Input: part model. Units: mm. Frame: model coordinates. Give positions to 0.01 mm unless a question says otherwise; leave off trailing zeros. Order: outer loops, then holes, each group sorted by start corner. A loop starts at its lowest first (then second) coordinate and runs counter-clockwise, first axis right, second up. Notation, with made-up numbers: (-28, 1.25) - (-16, 1.25) arc R19 cw to (-16, 15.25) - close; hole circle Ø8 at (80.5, 10.25). An arc over 180 degrees is marked (long way). Use a Markdown table: item, result.
Autodesk Inventor part; units mm, degrees
ref_plane "YZ Plane" through (0, 0, 0) normal (1, 0, 0) x (0, 1, 0)
ref_plane "XZ Plane" through (0, 0, 0) normal (0, 1, 0) x (-1, 0, 0)
ref_plane "XY Plane" through (0, 0, 0) normal (0, 0, 1) x (1, 0, 0)
sketch "Sketch2" plane through (0, 0, 0) normal (0, 0, 1) x (1, 0, 0)
  line L0 (0, 0) -> (-9.9, 0)
  line L1 (-4.95, 0) -> (-4.95, 2.5)
  line L2 (-4.95, 0) -> (-2.45, 0) construction
  circle A0 centre (-4.95, 5) radius 2.5
  line L3 (-4.95, 7.5) -> (32.05, 7.5) construction
  line L4 (0, 44.5) -> (0, 0)
  line L5 (0, 0) -> (-9.9, 0)
  line L6 (-9.9, 0) -> (-9.9, 44.5)
  line L7 (0, 45.5) -> (0, 0)
  line L8 (0, 0) -> (-9.9, 0)
  line L9 (-9.9, 0) -> (-9.9, 45.5)
  line L10 (-4.95, 7.5) -> (66.05, 7.5) construction
  line L11 (0, 0) -> (-9.9, 0)
  line L12 (-9.9, 0) -> (-9.9, 81)
  line L13 (-9.9, 81) -> (0, 81)
  line L14 (0, 81) -> (0, 0)
  dimension "d35" = 5
  dimension "d33" = 2.5
  dimension "d34" = 90
  dimension "d46" = 9.9
  dimension "d47" = 81
extrude "Extrusion6" add sketch "Sketch2" along normal blind 5
properties part number "Elbow_Cube_Holder_TestFit_V2"
1. Material intervals for line 1 along Y through (x, z) = (-4.95, 2.65); line 2 along X through (y, z) = (5, 1.35); line 3 along Y through (x, z) = (-7, 1.9), sorted ascending.
Response:
| item | result |
|---|---|
| line 1 | y = 0 to 2.5, 7.5 to 81 |
| line 2 | x = -9.9 to -7.45, -2.45 to 0 |
| line 3 | y = 0 to 3.57, 6.43 to 81 |
2. Section query A-A (x = -4.95). Return loops of the section in (y, z).
Response:
| item | result |
|---|---|
| outline | (0, 0) - (2.5, 0) - (2.5, 5) - (0, 5) - close; (7.5, 0) - (81, 0) - (81, 5) - (7.5, 5) - close |
3. Section query B-B (y = 6.5). Return loops of the section in (x, z), then the cut area to 3 significant figures.
Response:
| item | result |
|---|---|
| outline | (-9.9, 0) - (-6.95, 0) - (-6.95, 5) - (-9.9, 5) - close; (-2.95, 0) - (0, 0) - (0, 5) - (-2.95, 5) - close |
| area | 29.5 mm^2 |
4. Pin query (flat end, axial travel): pin 1 (5 mm diameter, centred on x = -6, y = 52, fed in from -Z). Return the tip coordinate at first contact, or that it passes through.
Response:
| item | result |
|---|---|
| pin 1 | stops at z = 0 |
5. Section query C-C (z = 3). Return loops of the section in (x, y).
Response:
| item | result |
|---|---|
| outline | (-9.9, 0) - (0, 0) - (0, 81) - (-9.9, 81) - close; hole circle Ø5 at (-4.95, 5) |
6. Mould query, pull axis Y, two halves, no side actions, for faces 1 (the face through (-2.565, 4.249, 2.465)), 2 (the face through (-5, 81, 2)), 3 (the face through (-9.9, 40, 2)). Classes: pulls with the +Y half, pulls with the -Y half, needs draft (parallel to the pull), parting line crosses it, or undercut.
Response:
| item | result |
|---|---|
| face 1 | undercut |
| face 2 | pulls with the +Y half |
| face 3 | needs draft |
